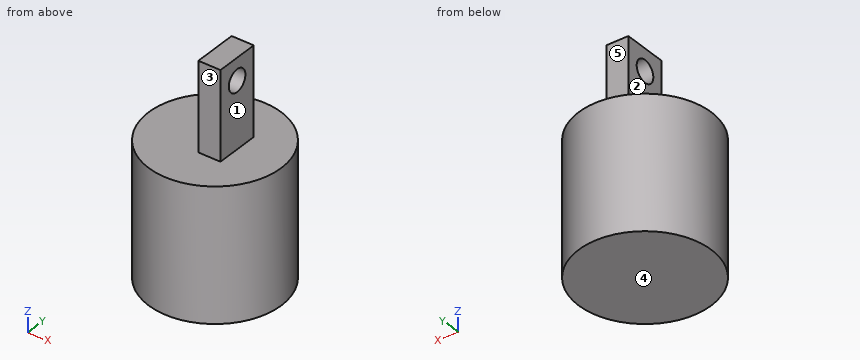
from build123d import *

# Parameters (mm, degrees)
SKETCH003_R  = 15
PAD003_DEPTH = 30
SKETCH004_W  = 5
SKETCH004_H  = 10
PAD004_DEPTH = 20
SKETCH005_R  = 2.5
POCKET_DEPTH = 20.001


with BuildPart() as part:
    # Sketch003 → Pad003 (new body)
    with BuildSketch(Plane.XY):
        Circle(SKETCH003_R)
    extrude(amount=PAD003_DEPTH)

    # Sketch004 (on Face3 of Pad003) → Pad004 (join)
    with BuildSketch(Plane.XY.offset(30)):
        with Locations((2.5, 0)):
            Rectangle(SKETCH004_W, SKETCH004_H)
    extrude(amount=PAD004_DEPTH)

    # Sketch005 (on Face6 of Pad004) → Pocket (cut, through all)
    with BuildSketch(Plane.YZ.offset(5)):
        with Locations((0, 45)):
            Circle(SKETCH005_R)
    extrude(amount=-POCKET_DEPTH, mode=Mode.SUBTRACT)


solid = part.part
Design review of the part built by this model. Coordinates are the model's own, in mm. Face numbers are marked on the shaded views. A direction names the side the tool comes from. Round coordinates to 2 decimals unless told otherwise and drop trailing zeros. Write each loop counter-clockwise with the first axis right and the second up, starting at its lowest first coordinate (ties: lowest second). Pieces come first, ordered by that corner, then holes. Notation, with made-up numbers: (-30.5, 1) - (17.5, 1) arc R30 cw to (17.5, 36) - close; hole circle Ø8 at (-14.75, 38.25). An arc over 180 degrees is marked (long way). Use a Markdown table: item, result. Add a question column.
1. We need section C-C (x = -12). State the section outline as (y, z) points.
2. We need section B-B (z = 45). State the section outline as (x, y) points.
3. Clearance check with flat-ended pins moving along their axes: pin 1 (5 mm diameter, centred on y = 0, z = 39.5, fed in from +X); pin 2 (11 mm diameter, centred on y = 0, z = 39.5, fed in from -X); pin 3 (3 mm diameter, centred on x = -1.5, z = 14, fed in from +Y); pin 4 (6 mm diameter, centred on x = -10, z = 12, fed in from -Y). State where each tip first meets the part, or that it passes through.
4. For the marked faces 1, 2, 3, 4 and 5, list the 3-axis set-ups (+Z, -Z, +X, -X, +Y, -Y) from which the entire face can be reached by the end or side of a thin tool; tool diameter is ignored.
5. We need section A-A (y = 0). State the section outline as (x, z) points, then the cut area to 3 significant figures.
6. We need section D-D (y = 3.75). State the section outline as (x, z) points.
7. Wall thickness on probe 1 along Z at (x, y) = (1.45, 0); probe 2 along Z at (x, y) = (-4.5, 1.5); probe 3 along Y at (x, z) = (5.75, 27.5): over which ranges is each line inside the solid? List them lowest first.
Output:
| question | item | result |
|---|---|---|
| 1 | outline | (-9, 0) - (9, 0) - (9, 30) - (-9, 30) - close |
| 2 | outline | (0, -5) - (5, -5) - (5, -2.5) - (0, -2.5) - close; (0, 2.5) - (5, 2.5) - (5, 5) - (0, 5) - close |
| 3 | pin 1 | stops at x = 5 |
| 3 | pin 2 | stops at x = 0 |
| 3 | pin 3 | stops at y = 15 |
| 3 | pin 4 | stops at y = -13.27 |
| 4 | face 1 | +Z, +X, +Y, -Y |
| 4 | face 2 | +Z, -X, +Y, -Y |
| 4 | face 3 | +Z, +X, -X, -Y |
| 4 | face 4 | -Z, +X, -X, +Y, -Y |
| 4 | face 5 | +Z, +X, -X, +Y |
| 5 | outline | (-15, 0) - (15, 0) - (15, 30) - (5, 30) - (5, 42.5) - (0, 42.5) - (0, 30) - (-15, 30) - close; (0, 47.5) - (5, 47.5) - (5, 50) - (0, 50) - close |
| 5 | area | 975 mm2 |
| 6 | outline | (-14.52, 0) - (14.52, 0) - (14.52, 30) - (5, 30) - (5, 50) - (0, 50) - (0, 30) - (-14.52, 30) - close |
| 7 | probe 1 | z = 0 to 42.5, 47.5 to 50 |
| 7 | probe 2 | z = 0 to 30 |
| 7 | probe 3 | y = -13.85 to 13.85 |
